from build123d import *

# Parameters (mm, degrees)
SKETCH1_W           = 7
SKETCH1_H           = 7
BOSS_EXTRUDE1_DEPTH = 5
SKETCH4_R           = 1.65
CUT_EXTRUDE4_DEPTH  = 4
SKETCH6_R           = 1.65
CUT_EXTRUDE6_DEPTH  = 4
SKETCH6_4_R         = 1.65
BOSS_EXTRUDE2_DEPTH = 1.6


with BuildPart() as part:
    # Sketch1 → Boss-Extrude1 (new body)
    with BuildSketch(Plane(origin=(0, 0, 0), x_dir=(1, 0, 0), z_dir=(0, 1, 0))):
        with Locations((-0.67779661, -2.128287226)):
            Rectangle(SKETCH1_W, SKETCH1_H)
    extrude(amount=BOSS_EXTRUDE1_DEPTH)

    # Sketch4 → Cut-Extrude4 (cut)
    with BuildSketch(Plane(origin=(0, 5, 0), x_dir=(1, 0, 0), z_dir=(0, 1, 0))):
        Polygon((-1.416005829, 0.916524834), (-3.661371426, -1.328840764), (-2.839510577, -4.396067211), (0.22771587, -5.21792806), (2.473081468, -2.972562463), (1.651220618, 0.094663984), align=None)
        with Locations((-0.594144979, -2.150701613)):
            Circle(SKETCH4_R, mode=Mode.SUBTRACT)
    extrude(amount=-CUT_EXTRUDE4_DEPTH, mode=Mode.SUBTRACT)

    # Sketch6 → Cut-Extrude6 (cut)
    with BuildSketch(Plane(origin=(0, 5, 0), x_dir=(1, 0, 0), z_dir=(0, 1, 0))):
        with Locations((-0.594144979, -2.150701613)):
            Circle(SKETCH6_R)
    extrude(amount=-CUT_EXTRUDE6_DEPTH, mode=Mode.SUBTRACT)

    # Sketch6_4 → Boss-Extrude2 (add)
    with BuildSketch(Plane(origin=(0, 5, 0), x_dir=(1, 0, 0), z_dir=(0, 1, 0))):
        Polygon((1.651220618, 0.094663984), (-1.416005829, 0.916524834), (-3.661371426, -1.328840764), (-2.839510577, -4.396067211), (0.22771587, -5.21792806), (2.473081468, -2.972562463), align=None)
        with Locations((-0.594144979, -2.150701613)):
            Circle(SKETCH6_4_R, mode=Mode.SUBTRACT)
    extrude(amount=-BOSS_EXTRUDE2_DEPTH)


solid = part.part
The listing builds one solid part. Answer for the finished solid, in the listing's coordinates (mm). A direction names the side the tool comes from. Round coordinates to 2 decimals unless told otherwise and drop trailing zeros. Loops run counter-clockwise (first coordinate to the right, second up) from the corner with the lowest first, then second, coordinate; pieces in that order, holes last. Notation, with made-up numbers: M 7.5,-27 L 19.5,-27 A23 cw 19.5,4 Z; hole C -22,57 d6. An arc over 180 degrees is marked long. Write each question's results on one line, items separated by ' | '. Start each with the question number.
1) Find section C-C on x = -0.25. Write down the section's boundary in (y, z).
2) Find section B-B on z = 4. Write down the section's boundary in (x, y), plus the area to 3 significant figures.
3) Which of the six approach directions +Z, -Z, +X, -X, +Y, -Y give full straight-line access (tool end or side, diameter ignored) to faces 1 (the flat face through (0.14, 2.22, -0.5)), 2 (the cylindrical face through (0.293, 4.211, 0.759)), 3 (the flat face through (-1, 2, -1.372))?
4) Find section A-A on y = 1.1. Write down the section's boundary in (x, z).
5) Straight lines are drawn through the part: probe 1 along Y at (x, z) = (-2.75, 0.75); probe 2 along X at (y, z) = (4.3, 2.25); probe 3 along Y at (x, z) = (-1.5, 2). For each, find the intervals that lie inside material, in ascending order.
6) Find section D-D on x = 2.25. Write down the section's boundary in (y, z), plus the area to 3 significant figures.
7) Determine the mould class of faces 4 (the flat face through (-2, 5, 1)), 5 (the flat face through (1, 3.4, 3)), 6 (the flat face through (-1, 2, 5.628)) for opening direction Y: pulls with the +Y half, pulls with the -Y half, needs draft (parallel to the pull), parting line crosses it, or undercut.
Final values:
1) outline: M 0,-1.37 L 5,-1.37 L 5,0.54 L 3.4,0.54 L 3.4,-0.6 L 1,-0.6 L 1,5.09 L 3.4,5.09 L 3.4,3.76 L 5,3.76 L 5,5.63 L 0,5.63 Z
2) outline: M -4.18,0 L 2.82,0 L 2.82,5 L -4.18,5 Z; hole M -2.95,1 L 1.45,1 L 1.45,3.4 L -2.95,3.4 Z | area: 24.5 mm²
3) face 1: none | face 2: +Y | face 3: -Z, +X, -X, +Y, -Y
4) outline: M -4.18,-1.37 L 2.82,-1.37 L 2.82,5.63 L -4.18,5.63 Z; hole M -3.66,1.33 L -1.42,-0.92 L 1.65,-0.09 L 2.47,2.97 L 0.23,5.22 L -2.84,4.4 Z
5) probe 1: 0 to 1, 3.4 to 5 | probe 2: -4.18 to -2.24, 1.05 to 2.82 | probe 3: 0 to 1
6) outline: M 0,-1.37 L 5,-1.37 L 5,5.63 L 0,5.63 Z; hole M 1,2.14 L 3.4,2.14 L 3.4,3.2 L 1,3.2 Z | area: 32.5 mm²
7) face 4: pulls with the +Y half | face 5: undercut | face 6: needs draft
